from build123d import *

# Parameters (mm, degrees)
F1_DEPTH = 12.7
F2_DEPTH = 12.7
F3_DEPTH = 12.7
F4_W     = 6.35
F4_H     = 25.4
F5_DEPTH = 62.464519896


# Not quite as in the source:
# - a feature names something its author has since deleted; it is built from what else it names


with BuildPart() as f1:
    # F0 (on Top) → F1 (new body, symmetric)
    with BuildSketch(Plane.XY):
        with BuildLine():
            ThreePointArc((-35.5333842184, -13.7473126824), (0.1257546156, 38.0997924637), (35.4418604651, -13.9815781216))
            ThreePointArc((35.4418604651, -13.9815781216), (36.7563215678, -25.7870785948), (47.2558139535, -31.3421041622))
            Line((47.2558139535, -31.3421041622), (104.4058139535, -31.3421041622))
            ThreePointArc((104.4058139535, -31.3421041622), (110.669864998, -28.7474492641), (113.264519896, -22.4833982196))
            Line((113.264519896, -22.4833982196), (113.264519896, 44.45))
            Line((113.264519896, 44.45), (106.914519896, 44.45))
            Line((106.914519896, 44.45), (106.914519896, -22.4833982196))
            ThreePointArc((106.914519896, -22.4833982196), (106.1797369375, -24.2573212036), (104.4058139535, -24.9921041622))
            Line((104.4058139535, -24.9921041622), (47.2558139535, -24.9921041622))
            ThreePointArc((47.2558139535, -24.9921041622), (42.0060677606, -22.2145913785), (41.3488372093, -16.3118411419))
            ThreePointArc((41.3488372093, -16.3118411419), (43.6678274818, -8.3020083729), (44.45, 0))
            ThreePointArc((44.45, 0), (31.4308965011, 31.4308963464), (2.188e-07, 44.45))
            ThreePointArc((2.188e-07, 44.45), (-31.4308963464, 31.4308965011), (-44.45, 0))
            ThreePointArc((-44.45, 0), (-43.6949916081, -8.157831107), (-41.4556149214, -16.0385314629))
            ThreePointArc((-41.4556149214, -16.0385314629), (-41.4024515906, -16.1752744115), (-41.3488372093, -16.3118411419))
            ThreePointArc((-41.3488372093, -16.3118411419), (-38.7334132864, -21.806540193), (-35.3920150029, -26.8925226418))
            ThreePointArc((-35.3920150029, -26.8925226418), (-30.9431194568, -27.499629239), (-30.3360128596, -23.0507336929))
            ThreePointArc((-30.3360128596, -23.0507336929), (-33.2615811181, -18.581636675), (-35.5333842184, -13.7473126825))
        make_face()
    extrude(amount=F1_DEPTH, both=True)

    # F0 (on Top) → F2 (join, symmetric)
    with BuildSketch(Plane.XY):
        with BuildLine():
            Line((44.45, 0), (44.45, 44.45))
            Line((44.45, 44.45), (2.188e-07, 44.45))
            ThreePointArc((2.188e-07, 44.45), (31.4308965011, 31.4308963464), (44.45, 0))
        make_face()
    extrude(amount=F2_DEPTH, both=True)

    # F0 (on Top) → F3 (join, symmetric)
    with BuildSketch(Plane.XY):
        with BuildLine():
            Line((-44.45, 44.45), (-44.45, 0))
            ThreePointArc((-44.45, 0), (-31.4308963464, 31.4308965011), (2.188e-07, 44.45))
            Line((2.188e-07, 44.45), (-44.45, 44.45))
        make_face()
    extrude(amount=F3_DEPTH, both=True)

    # F4 (on face) → F5 (join, through all)
    with BuildSketch(Plane(origin=(106.914519896, 0, 0), x_dir=(0, -1, 0), z_dir=(-1, 0, 0))):
        with Locations((-41.275, 0)):
            Rectangle(F4_W, F4_H)
    extrude(amount=F5_DEPTH)


solid = f1.part
Here's how the part is built. I have some questions about the finished solid (model axes, mm). A direction names the side the tool comes from. Coordinates: 2 decimals unless noted, no trailing zeros. Loops run counter-clockwise (first coordinate to the right, second up) from the corner with the lowest first, then second, coordinate; pieces in that order, holes last. Notation, with made-up numbers: (-3, 0) -> (52, 0) arc R20 cw to (52, 28) -> close; hole circle Ø6 at (18.5, 28). An arc over 180 degrees is marked (long way). Use one line per item in the form item = value. Start each with the question number.
(1) On a 3-axis mill with a long thin cutter (end or side, diameter ignored), from which of +Z, -Z, +X, -X, +Y, -Y can I reach the whole of each face in a straight line? I mean faces 1 (the face through (35, 18, -12.7)), 2 (the face through (44.45, 19, 0)). Say none if no direction works.
(2) Will these pins go through, and if not, where does the flat tip stop? pin 1 (8 mm diameter, centred on y = -15, z = 0.5, fed in from -X); pin 2 (1 mm diameter, centred on x = 6.5, z = 1, fed in from -Y).
(3) If we section it at D-D (y = 25.5): Please give me the cut outline in (x, z), then the cut area to 3 significant figures.
(4) We'd pull the mould along X, two halves only. Please class faces 3 (the face through (36, 44.45, 0)), 4 (the face through (113.265, 11, 0)), 5 (the face through (-31, -27.54, 0.18)): pulls with the +X half, pulls with the -X half, needs draft (parallel to the pull), parting line crosses it, or undercut.
(5) If we section it at B-B (y = 2.5): Please give me the cut outline in (x, z).
(6) Please list where these lines run through material, in increasing order: line 1 along X through (y, z) = (-15, -4.25); line 2 along Y through (x, z) = (56.5, 2.75); line 3 along X through (y, z) = (16, 11.25).
(7) If we section it at C-C (z = 7.25): Please give me the cut outline in (x, y) (3 decimals), then the cut area to 3 significant figures.
(8) If we section it at A-A (x = 58): Please give me the cut outline in (y, z).
Verdict:
q1.face_1 = -Z, +X, -X, +Y, -Y
q1.face_2 = +Z, -Z
q2.pin_1 = -43.07
q2.pin_2 = 37.45
q3.outline = (-44.45, -12.7) -> (-28.31, -12.7) -> (-28.31, 12.7) -> (-44.45, 12.7) -> close; (28.31, -12.7) -> (44.45, -12.7) -> (44.45, 12.7) -> (28.31, 12.7) -> close; (106.91, -12.7) -> (113.26, -12.7) -> (113.26, 12.7) -> (106.91, 12.7) -> close
q3.area = 981 mm²
q4.face_3 = needs draft
q4.face_4 = pulls with the +X half
q4.face_5 = undercut
q5.outline = (-44.45, -12.7) -> (-38.02, -12.7) -> (-38.02, 12.7) -> (-44.45, 12.7) -> close; (38.02, -12.7) -> (44.45, -12.7) -> (44.45, 12.7) -> (38.02, 12.7) -> close; (106.91, -12.7) -> (113.26, -12.7) -> (113.26, 12.7) -> (106.91, 12.7) -> close
q6.line_1 = -41.84 to -35.02, 35.09 to 41.84, 106.91 to 113.26
q6.line_2 = -31.34 to -24.99, 38.1 to 44.45
q6.line_3 = -44.45 to -34.58, 34.58 to 44.45, 106.91 to 113.26
q7.outline = (-44.45, 0) arc R44.45 ccw to (-41.456, -16.039) arc R44.45 ccw to (-41.349, -16.312) arc R44.45 ccw to (-35.392, -26.893) arc R3.175 ccw to (-30.336, -23.051) arc R38.1 cw (long way) to (35.442, -13.982) arc R12.7 ccw to (47.256, -31.342) -> (104.406, -31.342) arc R8.859 ccw to (113.265, -22.483) -> (113.265, 44.45) -> (-44.45, 44.45) -> close; hole (41.349, -16.312) arc R6.35 ccw to (47.256, -24.992) -> (104.406, -24.992) arc R2.509 ccw to (106.915, -22.483) -> (106.915, 38.1) -> (44.45, 38.1) -> (44.45, 0) arc R44.45 cw to start
q7.area = 3,320 mm²
q8.outline = (-31.34, -12.7) -> (-24.99, -12.7) -> (-24.99, 12.7) -> (-31.34, 12.7) -> close; (38.1, -12.7) -> (44.45, -12.7) -> (44.45, 12.7) -> (38.1, 12.7) -> close
